Source: CAD feature listing. Evaluate the final solid. Frame: model axes, mm. Coordinates: 2 decimals unless noted, no trailing zeros. Loops run counter-clockwise (first coordinate to the right, second up) from the corner with the lowest first, then second, coordinate; pieces in that order, holes last. Notation, with made-up numbers: M 81.5,74 L 101.5,74 A31 ccw 101.5,108 Z; hole C -16,9.25 d2. An arc over 180 degrees is marked long. Write each question's results on one line, items separated by ' | '. Start each with the question number.
from build123d import *

# Parameters (mm, degrees)
F1_DEPTH = 5


with BuildPart() as f1:
    # F0 (on Top) → F1 (new body)
    with BuildSketch(Plane.XY):
        with BuildLine():
            ThreePointArc((-7.531189, 65.674413), (-13.478061, 64.012162), (-19.424933, 65.674413))
            ThreePointArc((-19.424933, 65.674413), (-27.691208, 65.630451), (-30.896061, 58.010598))
            Line((-30.896061, 58.010598), (-30.628454, 56.988378))
            Line((-30.628454, 56.988378), (-23.195385, 28.595213))
            Line((-23.195385, 28.595213), (-13.195385, 28.595213))
            Line((-13.195385, 28.595213), (-3.195385, 28.595213))
            Line((-3.195385, 28.595213), (3.75462, 57.24662))
            Line((3.75462, 57.24662), (3.93994, 58.010598))
            ThreePointArc((3.93994, 58.010598), (0.735086, 65.630451), (-7.531189, 65.674413))
        make_face()
    extrude(amount=F1_DEPTH)


solid = f1.part
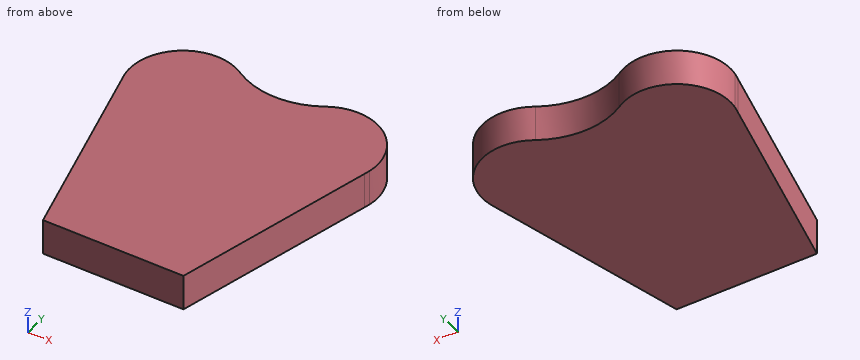
Item 1: Cut plane C-C (x = -18). Output: boundary loops of the cut face in (y, z), then the cut area to 3 significant figures.
Item 2: Cut plane D-D (y = 50). Output: boundary loops of the cut face in (x, z).
Item 3: First-contact query: pin 1 Ø2 at (y, z) = (48.5, 1) entering from +X. Flat tip, straight axial feed; report the tip coordinate or a pass-through.
Item 4: Cut plane B-B (y = 64.5). Output: boundary loops of the cut face in (x, z).
Item 5: Line query: probe 1 along X at (y, z) = (58, 4.4); probe 2 along X at (y, z) = (65.5, 2.45); probe 3 along Y at (x, z) = (-13.5, 3.4). Output: solid intervals per line, ascending.
Item 6: Cut plane A-A (z = 4.45). Output: boundary loops of the cut face in (x, y).
Response values:
1) outline: M 28.6,0 L 64.94,0 L 64.94,5 L 28.6,5 Z | area: 182 mm2
2) outline: M -28.8,0 L 2,0 L 2,5 L -28.8,5 Z
3) pin 1: stops at x = 1.88
4) outline: M -29.02,0 L -16.79,0 L -16.79,5 L -29.02,5 Z; M -10.17,0 L 2.06,0 L 2.06,5 L -10.17,5 Z
5) probe 1: x = -30.89 to 3.94 | probe 2: x = -27.88 to -19.13, -7.83 to 0.92 | probe 3: y = 28.6 to 64.01
6) outline: M -30.9,58.01 L -30.63,56.99 L -23.2,28.6 L -3.2,28.6 L 3.75,57.25 L 3.94,58.01 A7.5 ccw -7.53,65.67 A11.47 cw -19.42,65.67 A7.5 ccw Z
